Verification items for the finished model (mm, model axes). Face numbers are marked on the shaded views. A direction names the side the tool comes from. Round coordinates to 2 decimals unless told otherwise and drop trailing zeros. Write each loop counter-clockwise with the first axis right and the second up, starting at its lowest first coordinate (ties: lowest second). Pieces come first, ordered by that corner, then holes. Notation, with made-up numbers: (60.5, 73.25) - (115.5, 73.25) arc R27 ccw to (115.5, 92.25) - close; hole circle Ø10 at (72.5, -18). An arc over 180 degrees is marked (long way). Write each question's results on one line, items separated by ' | '.
```python
from build123d import *

# Parameters (mm, degrees)
SKETCH1_R           = 7.9375
BOSS_EXTRUDE1_DEPTH = 0.381
BOSS_EXTRUDE2_DEPTH = 3.81
SKETCH3_R           = 6.35
CUT_EXTRUDE1_DEPTH  = 5.572


with BuildPart() as part:
    # Sketch1 → Boss-Extrude1 (new body, symmetric)
    with BuildSketch(Plane(origin=(0, 0, 0), x_dir=(1, 0, 0), z_dir=(0, 1, 0))):
        Circle(SKETCH1_R)
    extrude(amount=BOSS_EXTRUDE1_DEPTH, both=True)

    # Sketch2 → Boss-Extrude2 (add)
    with BuildSketch(Plane(origin=(0, 0.381, 0), x_dir=(1, 0, 0), z_dir=(0, 1, 0))):
        Polygon((-3.96875, -6.874076643), (3.96875, -6.874076643), (7.9375, 0), (3.96875, 6.874076643), (-3.96875, 6.874076643), (-7.9375, 0), align=None)
    extrude(amount=BOSS_EXTRUDE2_DEPTH)

    # Sketch3 → Cut-Extrude1 (cut, through all)
    with BuildSketch(Plane(origin=(0, 4.191, 0), x_dir=(1, 0, 0), z_dir=(0, 1, 0))):
        Circle(SKETCH3_R)
    extrude(amount=-CUT_EXTRUDE1_DEPTH, mode=Mode.SUBTRACT)


solid = part.part
```
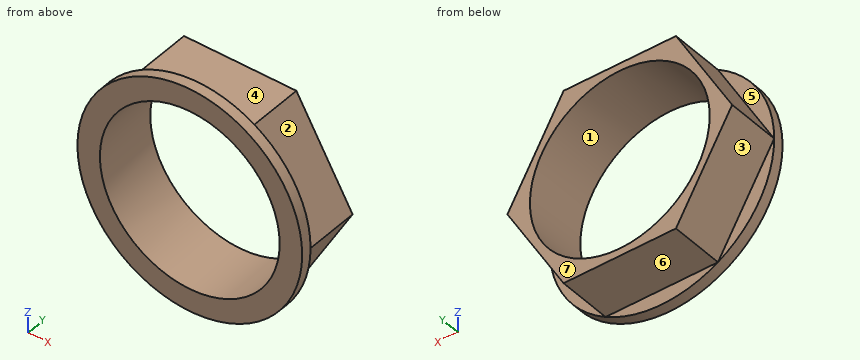
(1) Set-up check for the marked faces 4, 5, 6 and 7: record each of +Z, -Z, +X, -X, +Y, -Y from which the full face is reachable in a straight line by a thin tool's end or side.
Answer:
face 4: +Z, +X, -X, +Y | face 5: +Z, -X, +Y | face 6: -Z, +X, -X, +Y | face 7: +Z, -Z, +X, -X, +Y
(2) Section check C-C (z = -5). Record the cut outline in (x, y), plus the area to 3 significant figures.
Answer:
outline: (-6.16, -0.38) - (-3.91, -0.38) - (-3.91, 4.19) - (-5.05, 4.19) - (-5.05, 0.38) - (-6.16, 0.38) - close; (3.91, -0.38) - (6.16, -0.38) - (6.16, 0.38) - (5.05, 0.38) - (5.05, 4.19) - (3.91, 4.19) - close | area: 12.1 mm2
(3) Mould release check, pull along X, two halves, no side actions. Record for the marked faces 1, 2 and 3: released by +X, released by -X, zero draft, split by the parting line, or undercut.
Answer:
face 1: undercut | face 2: released by +X | face 3: released by -X
(4) Section check A-A (y = 0.7). Record the cut outline in (x, z), plus the area to 3 significant figures.
Answer:
outline: (-7.94, 0) - (-3.97, -6.87) - (3.97, -6.87) - (7.94, 0) - (3.97, 6.87) - (-3.97, 6.87) - close; hole circle Ø12.7 at (0, 0) | area: 37.0 mm2
(5) Section check B-B (x = 0). Record the cut outline in (y, z).
Answer:
outline: (-0.38, -7.94) - (0.38, -7.94) - (0.38, -6.87) - (4.19, -6.87) - (4.19, -6.35) - (-0.38, -6.35) - close; (-0.38, 6.35) - (4.19, 6.35) - (4.19, 6.87) - (0.38, 6.87) - (0.38, 7.94) - (-0.38, 7.94) - close
(6) Thickness scan on L1, parallel to Z at x = 0, y = 1.15; L2, parallel to X at y = -0.1, z = 1.75; L3, parallel to Z at x = -1.25, y = 1.7. Record the ranges inside material, lowest first.
Answer:
L1: -6.87 to -6.35, 6.35 to 6.87 | L2: -7.74 to -6.1, 6.1 to 7.74 | L3: -6.87 to -6.23, 6.23 to 6.87
(7) Go/stop test with flat-tipped pins: pin 1 Ø2 at (x, y) = (-5.5, 2) entering from +Z; pin 2 Ø1.5 at (x, y) = (4.5, 1.5) entering from +Z; pin 3 Ø1 at (y, z) = (2, 2.5) entering from +X. Record where each tip stops, or that it passes through.
Answer:
pin 1: z = 5.95 | pin 2: z = 6.87 | pin 3: x = 6.78
